```python
from build123d import *

# Parameters (mm, degrees)
EXTRUDE_THIN1_DEPTH = 100
CUT_EXTRUDE2_DEPTH  = 33.5
FILLET1_R           = 3
SKETCH6_W           = 108.670856817
SKETCH6_H           = 17.879774232
CUT_EXTRUDE3_DEPTH  = 166
BOSS_EXTRUDE1_DEPTH = 10
CUT_EXTRUDE4_DEPTH  = 27
SKETCH11_R          = 1.75
CUT_EXTRUDE5_DEPTH  = 5
SKETCH12_W          = 11.662154679
SKETCH12_H          = 21.882804931
BOSS_EXTRUDE2_DEPTH = 7.5
CUT_EXTRUDE7_DEPTH  = 5
FILLET5_R           = 12
SKETCH16_W          = 5
SKETCH16_H          = 3
BOSS_EXTRUDE3_DEPTH = 4


with BuildPart() as part:
    # Sketch1 → Extrude-Thin1 (new body)
    with BuildSketch(Plane(origin=(0, 0, 0), x_dir=(0, 0, -1), z_dir=(1, 0, 0))):
        with BuildLine():
            Line((45, -32), (45, -18))
            ThreePointArc((45, -18), (32.040658091, -6.957616726), (16.501342128, 0))
            ThreePointArc((16.501342128, 0), (0, 1.972757604), (-16.501342128, 0))
            ThreePointArc((-16.501342128, 0), (-32.040658091, -6.957616726), (-45, -18))
            Line((-45, -18), (-45, -32))
            Line((-45, -32), (-48, -32))
            Line((-48, -32), (-48, -16.88185814))
            ThreePointArc((-48, -16.88185814), (-34.099982932, -4.712774746), (-17.26768466, 2.901081048))
            ThreePointArc((-17.26768466, 2.901081048), (0, 4.972757604), (17.26768466, 2.901081048))
            ThreePointArc((17.26768466, 2.901081048), (34.099982932, -4.712774746), (48, -16.88185814))
            Line((48, -16.88185814), (48, -32))
            Line((48, -32), (45, -32))
        make_face()
    extrude(amount=EXTRUDE_THIN1_DEPTH)

    # Sketch5 → Cut-Extrude2 (cut, symmetric)
    with BuildSketch(Plane(origin=(0, 0, 0), x_dir=(1, 0, 0), z_dir=(0, 1, 0))):
        with BuildLine():
            Line((74.78082212, 3), (74.78082212, -3))
            add(Edge.make_bspline(
                [(74.78082212, -3), (97.634090292, -10.562952057), (100, -44)],
                knots=[0, 0, 0, 1, 1, 1], degree=2))
            Line((100, -44), (100, 44))
            add(Edge.make_bspline(
                [(74.78082212, 3), (97.634090292, 10.562952057), (100, 44)],
                knots=[0, 0, 0, 1, 1, 1], degree=2))
        make_face()
    extrude(amount=CUT_EXTRUDE2_DEPTH, both=True, mode=Mode.SUBTRACT)

    # Fillet1
    fillet1_edges = [part.edges().sort_by_distance(p)[0] for p in [
        (50, -16.88185814, -48),
        (50, -16.88185814, 48),
        (74.78082212, 3.409765032, 3),
        (74.78082212, 3.409765032, -3),
        (46.328171757, 2.901081048, -17.26768466),
        (46.328171757, 2.901081048, 17.26768466),
    ]]
    fillet(fillet1_edges, radius=FILLET1_R)

    # Sketch6 → Cut-Extrude3 (cut)
    with BuildSketch(Plane(origin=(0, 0, -48), x_dir=(-1, 0, 0), z_dir=(0, 0, -1))):
        with Locations((-40.664571591, -32.939887116)):
            Rectangle(SKETCH6_W, SKETCH6_H)
    extrude(amount=-CUT_EXTRUDE3_DEPTH, mode=Mode.SUBTRACT)

    # Sketch8 → Boss-Extrude1 (add, symmetric)
    with BuildSketch(Plane.XY):
        Polygon((0, 1.972757604), (-2.848910504, -18), (7.151089496, -18), (15, 1.972757604), align=None)
    extrude(amount=BOSS_EXTRUDE1_DEPTH, both=True)

    # Sketch10 → Cut-Extrude4 (cut)
    with BuildSketch(Plane.XY.offset(10)):
        with BuildLine():
            Line((-0.348910504, -18), (3.987157996, -18))
            ThreePointArc((3.987157996, -18), (1.819123746, -14.255159652), (-0.348910504, -18))
        make_face()
    extrude(amount=-CUT_EXTRUDE4_DEPTH, mode=Mode.SUBTRACT)

    # Sketch11 → Cut-Extrude5 (cut)
    with BuildSketch(Plane(origin=(0, 0, -48), x_dir=(-1, 0, 0), z_dir=(0, 0, -1))):
        with Locations(Location((-95, -19, 0), (0, 0, 34.849904579))):
            Circle(SKETCH11_R)
    cut_extrude5 = extrude(amount=-CUT_EXTRUDE5_DEPTH, mode=Mode.SUBTRACT)

    # Mirror1: Cut-Extrude5 across plane
    add(cut_extrude5.mirror(Plane.XY), mode=Mode.SUBTRACT)

    # Sketch12 → Boss-Extrude2 (add, symmetric)
    with BuildSketch(Plane.XY):
        with Locations((68.949744781, -8.968644861)):
            Rectangle(SKETCH12_W, SKETCH12_H)
    extrude(amount=BOSS_EXTRUDE2_DEPTH, both=True)

    # Sketch15 → Cut-Extrude7 (cut)
    with BuildSketch(Plane(origin=(0, 0, -48), x_dir=(-1, 0, 0), z_dir=(0, 0, -1))):
        Polygon((-95, -24), (0, -18.860125055), (0, -26.57204687), align=None)
    cut_extrude7 = extrude(amount=-CUT_EXTRUDE7_DEPTH, mode=Mode.SUBTRACT)

    # Mirror2: Cut-Extrude7 across plane
    add(cut_extrude7.mirror(Plane.XY), mode=Mode.SUBTRACT)

    # Fillet5
    # the kernel refuses this fillet: 12 mm, written as the material it takes off along each edge
    with BuildSketch(Plane(origin=(0, -18.860125055, 76.420758066), x_dir=(0, 1, 0), z_dir=(0, 0, -1))) as fillet5_piece_1:
        with BuildLine():
            CenterArc((FILLET5_R * 0.947358602211, FILLET5_R), FILLET5_R, 183.096908366, 86.903091634)
            Line((-FILLET5_R * 0.0511809847104, FILLET5_R * 0.945975067318), (0, 0))
            Line((0, 0), (FILLET5_R * 0.947358602211, 0))
        make_face()
    extrude(amount=59.841516133, mode=Mode.SUBTRACT)
    with BuildSketch(Plane(origin=(0, -18.860125055, -76.420758066), x_dir=(0, 1, 0), z_dir=(0, 0, 1))) as fillet5_piece_2:
        with BuildLine():
            CenterArc((FILLET5_R * 0.947358602211, -FILLET5_R), FILLET5_R, 90, 86.903091634)
            Line((-FILLET5_R * 0.0511809847104, -FILLET5_R * 0.945975067318), (0, 0))
            Line((0, 0), (FILLET5_R * 0.947358602211, 0))
        make_face()
    extrude(amount=59.841516133, mode=Mode.SUBTRACT)

    # Sketch16 → Boss-Extrude3 (add)
    with BuildSketch(Plane.XZ.offset(32)):
        with Locations((97.5, -46.5)):
            Rectangle(SKETCH16_W, SKETCH16_H)
    boss_extrude3 = extrude(amount=BOSS_EXTRUDE3_DEPTH)

    # Mirror3: Boss-Extrude3 across plane
    add(boss_extrude3.mirror(Plane.XY))


solid = part.part
```
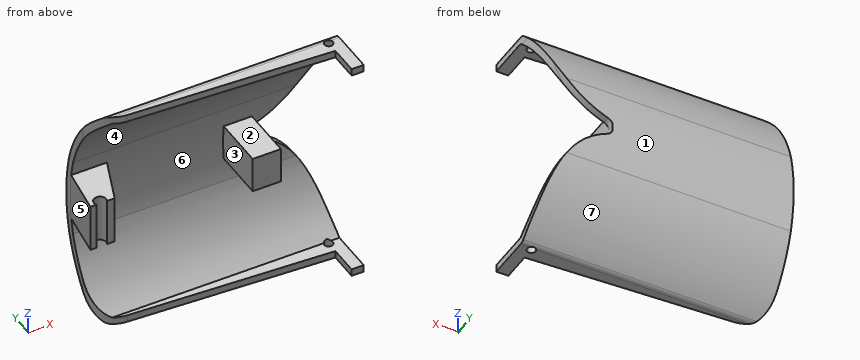
Design review of the part built by this model. Coordinates are the model's own, in mm. Face numbers are marked on the shaded views. A direction names the side the tool comes from. Coordinates: 2 decimals unless noted, no trailing zeros. Loops run counter-clockwise (first coordinate to the right, second up) from the corner with the lowest first, then second, coordinate; pieces in that order, holes last.
Q1. For pin 1 (12 mm diameter, centred on x = 14, z = -19.5, fed in from -Y); pin 2 (3.5 mm diameter, centred on x = 69, y = -7.5, fed in from -Z); pin 3 (8 mm diameter, centred on x = 59, z = 7.5, fed in from +Y), all flat-tipped, find the tip position at first contact; note any pin that passes through.
Reported:
pin 1: stops at y = -3.37
pin 2: stops at z = -40.29
pin 3: stops at y = 4.89
Q2. To check wall thickness, follow line 1 (Z direction, x = 71, y = -21.5); line 2 (Z direction, x = 61, y = -5); line 3 (X direction, y = 0.5, z = -6). State the ranges of each line that lie inside material, in increasing order.
Reported:
line 1: z = -48 to -45, 45 to 48
line 2: z = -34.54 to -28.71, 28.71 to 34.54
line 3: x = -0.21 to 14.42, 63.12 to 74.78
Q3. We need section A-A on y = -27. State the section outline as (x, z) points.
Reported:
outline: (95, -48) - (100, -48) - (100, -45) - (95, -45) - close; (95, 45) - (100, 45) - (100, 48) - (95, 48) - close
Q4. Tool access review of the marked faces 1, 2, 3 and 4: name each direction out of +Z, -Z, +X, -X, +Y, -Y from which nothing blocks a thin tool from reaching the whole face with its end or side.
Reported:
face 1: +X, -X, +Y
face 2: +X, -Y
face 3: -Y
face 4: +X, -X, -Y
Q5. We need section B-B on x = 36.5. State the section outline as (y, z) points.
Reported:
outline: (-20.83, -48) - (-18, -48) arc R3 ccw to (-16.02, -47.25) arc R63 ccw to (2.9, -17.27) arc R73 ccw to (2.9, 17.27) arc R63 ccw to (-16.02, 47.25) arc R3 ccw to (-18, 48) - (-20.83, 48) - (-20.83, 45) - (-18, 45) arc R60 cw to (0, 16.5) arc R70 cw to (0, -16.5) arc R60 cw to (-18, -45) - (-20.83, -45) - close
Q6. The part is to be moulded in two halves that separate along Z. For the marked faces 5, 6 and 7, say which applies: +Z half, -Z half, draft (parallel to the pull), parting line (faces both ways), or undercut.
Reported:
face 5: draft
face 6: undercut
face 7: -Z half
